The model under review builds one solid part; all positions refer to its coordinate system, in mm. A direction names the side the tool comes from. Round coordinates to 2 decimals unless told otherwise and drop trailing zeros. Loops run counter-clockwise (first coordinate to the right, second up) from the corner with the lowest first, then second, coordinate; pieces in that order, holes last. Notation, with made-up numbers: (51.5, -16) -> (55.5, -16) arc R24 ccw to (55.5, 23) -> close; hole circle Ø6 at (57, -12). An arc over 180 degrees is marked (long way). Use a Markdown table: item, result. Add a question column.
1) Mouldability with a two-part tool opening along Z and no side actions: class faces 5 (the cylindrical face through (8.728, 9.028, -60.264)), 6 (the cylindrical face through (5, 2, 0)), 7 (the cylindrical face through (19.014, 16.377, -42.653)) as released by +Z, released by -Z, zero draft, split by the parting line, or undercut.
2) Consider section B-B on x = 12.7. Give the boundary of the cut face in (y, z) (3 decimals), plus the area to 3 significant figures.
3) Consider section A-A on z = 8.75. Give the boundary of the cut face in (x, y).
4) Wall thickness on probe 1 along X at (y, z) = (10.5, -55); probe 2 along X at (y, z) = (12.25, -1.5); probe 3 along Y at (x, z) = (-12.7, -55.5) (3 decimals): over which ranges is each line inside the solid? List them lowest first.
5) Consider section C-C on z = -32.5. Give the boundary of the cut face in (x, y), plus the area to 3 significant figures.
6) Consider section D-D on x = 5. State how many separate pieces and enclosed holes the cut face has, plus the area to 3 significant figures.
7) Insertion check: pin 1 (1 mm diameter, centred on x = -15.5, z = -24, fed in from +Y); pin 2 (2 mm diameter, centred on x = 14, y = 17.5, fed in from +Z); pin 3 (4.5 mm diameter, centred on x = -2.5, y = 2, fed in from -Z); pin 4 (8 mm diameter, centred on x = -4.5, z = -44, fed in from +Y). Each pin has a flat end and moves straight along its axis. Give the tip position at first contact, or say it passes through.
8) For faces 1 (the flat face through (19, 15, 13)), 2 (the flat face through (0, 14.175, -56)), 3 (the cylindrical face through (-15.27, 2.46, -22.47)), 4 (the flat face through (13, 5, 10)), list the 3-axis set-ups (+Z, -Z, +X, -X, +Y, -Y) from which the entire face can be reached by the end or side of a thin tool; tool diameter is ignored.
from build123d import *

# Parameters (mm, degrees)
MAIN_DEPTH                      = 61.25
FRONT_CONGE_R                   = 3
ESQUISSE11_W                    = 2
ESQUISSE11_H                    = 15
DSUB_EXTRUSION_ATTACHMENT_DEPTH = 15
ESQUISSE12_W                    = 40
ESQUISSE12_H                    = 15
ESQUISSE12_R                    = 1.35
ESQUISSE12_W_2                  = 16
ESQUISSE12_H_2                  = 7
DSUB_EXTRUSION_DEPTH            = 15
DSUB_FRONT_HOLE_DEPTH           = 5.5
ESQUISSE14_R                    = 4.3
BOTTOM_HOLE_DEPTH               = 2
SKETCH7_W                       = 36
SKETCH7_H                       = 10
DSUBBOTTOMHOLE_DEPTH            = 1
CONG_4_R                        = 10
BOTTOMSTOP_REACH                = 77.839
SKETCH4_W                       = 6.5
SKETCH4_H                       = 7
FILLET1_R                       = 1
SKETCH5_W                       = 16
SKETCH5_H                       = 12
CUT_EXTRUDE1_DEPTH              = 14.175
SKETCH6_R                       = 1.25
FIXHOLE_DEPTH                   = 68.465268843
LPATTERN1_COUNT                 = 8
LPATTERN1_PITCH                 = 10
LPATTERN1_COUNT_DIR2            = 4
LPATTERN1_PITCH_DIR2            = 10


with BuildPart() as part:
    # Esquisse1 → Main (new, symmetric)
    with BuildSketch(Plane.XY):
        Polygon((18, 15), (20, 15), (20, 0), (-20, 0), (-20, 15), (-18, 15), (-18, 5), (-8, 5), (-8, 4), (8, 4), (8, 5), (18, 5), align=None)
    extrude(amount=MAIN_DEPTH, both=True)

    # Front Conge
    # the kernel refuses this fillet: 3 mm, written as the material it takes off along each edge
    with BuildSketch(Plane(origin=(18, 5, 61.25), x_dir=(1, 0, 0), z_dir=(0, 1, 0)), Plane(origin=(-18, 22.071067812, 61.25), x_dir=(-1, 0, 0), z_dir=(0, -1, 0))) as front_conge_piece_1:
        with BuildLine():
            CenterArc((3, 2.828427125), FRONT_CONGE_R, 180, 70.528779366)
            Line((0, 2.828427125), (-0.06, 2.828427125))
            Line((-0.06, 2.828427125), (-0.06, 0))
            Line((-0.06, 0), (0, -0.06))
            ThreePointArc((0, -0.06), (1, -0.06), (1.98, -0.056568542))
            Line((1.98, -0.056568542), (2, 0))
        make_face()
    extrude(amount=17.071067812, mode=Mode.SUBTRACT)

    # Esquisse11 → DSub-Extrusion Attachment (add)
    with BuildSketch(Plane(origin=(0, 0, -46.25), x_dir=(-1, 0, 0), z_dir=(0, 0, -1))):
        with Locations((-19, 12.5)):
            Rectangle(ESQUISSE11_W, ESQUISSE11_H)
        with Locations((19, 12.5)):
            Rectangle(ESQUISSE11_W, ESQUISSE11_H)
    extrude(amount=DSUB_EXTRUSION_ATTACHMENT_DEPTH)

    # Esquisse12 → DSub-Extrusion (add)
    with BuildSketch(Plane(origin=(0, 0, -46.25), x_dir=(-1, 0, 0), z_dir=(0, 0, -1))):
        with Locations((0, 12.5)):
            Rectangle(ESQUISSE12_W, ESQUISSE12_H)
        with Locations((-12.7, 10.675)):
            Circle(ESQUISSE12_R, mode=Mode.SUBTRACT)
        with Locations((12.7, 10.675)):
            Circle(ESQUISSE12_R, mode=Mode.SUBTRACT)
        with Locations((0, 10.675)):
            Rectangle(ESQUISSE12_W_2, ESQUISSE12_H_2, mode=Mode.SUBTRACT)
    extrude(amount=DSUB_EXTRUSION_DEPTH)

    # Esquisse13 → DSub-Front Hole (cut)
    with BuildSketch(Plane.XY.offset(-46.25)):
        Polygon((-10, 17), (10, 17), (8.5, 5), (-8.5, 5), align=None)
    extrude(amount=-DSUB_FRONT_HOLE_DEPTH, mode=Mode.SUBTRACT)

    # Esquisse14 → Bottom Hole (cut)
    with BuildSketch(Plane(origin=(0, 0, -61.25), x_dir=(-1, 0, 0), z_dir=(0, 0, -1))):
        with Locations((-12.7, 10.675)):
            Circle(ESQUISSE14_R)
        with Locations((12.7, 10.675)):
            Circle(ESQUISSE14_R)
    extrude(amount=-BOTTOM_HOLE_DEPTH, mode=Mode.SUBTRACT)

    # Sketch7 → DSubBottomHole (cut)
    with BuildSketch(Plane(origin=(0, 5, 0), x_dir=(1, 0, 0), z_dir=(0, 1, 0))):
        with Locations((0, 41.25)):
            Rectangle(SKETCH7_W, SKETCH7_H)
    extrude(amount=-DSUBBOTTOMHOLE_DEPTH, mode=Mode.SUBTRACT)

    # Congé4
    # the kernel refuses this fillet: 10 mm, written as the material it adds along each edge
    with BuildSketch(Plane(origin=(-18, 15, -46.25), x_dir=(0, 1, 0), z_dir=(-1, 0, 0)), Plane(origin=(20, 15, -46.25), x_dir=(0, 1, 0), z_dir=(-1, 0, 0))) as cong_4_piece_1:
        with BuildLine():
            CenterArc((10, -8.660254038), CONG_4_R, 120, 60)
            Line((0, -8.660254038), (0, 0))
            Line((0, 0), (5, 0))
        make_face()
    extrude(amount=2)

    # BottomStop: up to this face of the body (flat: up to its plane)
    bottomstop_end = Plane(part.part.faces().sort_by_distance((20, 7.947826544, -2.383218252))[0])
    # Sketch4 → BottomStop (add, up to the picked face)
    with BuildSketch(Plane.ZY.offset(20), mode=Mode.PRIVATE) as bottomstop_sk1:
        with Locations((58, 3.5)):
            Rectangle(SKETCH4_W, SKETCH4_H)
    bottomstop_tool1 = split(extrude(bottomstop_sk1.sketch, amount=-BOTTOMSTOP_REACH, mode=Mode.PRIVATE), bisect_by=bottomstop_end, keep=Keep.BOTH, mode=Mode.PRIVATE)
    add(bottomstop_tool1.solids().sort_by(Axis((-20, 3.5, 58), (1, 0, 0)))[0])

    # Fillet1
    fillet1_edges = [part.edges().sort_by_distance(p)[0] for p in [
        (0, 4, 54.75),
        (0, 7, 54.75),
    ]]
    fillet(fillet1_edges, radius=FILLET1_R)

    # Sketch5 → Cut-Extrude1 (cut)
    with BuildSketch(Plane(origin=(0, 0, 0), x_dir=(-1, 0, 0), z_dir=(0, -1, 0))):
        with Locations((0, 55.25)):
            Rectangle(SKETCH5_W, SKETCH5_H)
    extrude(amount=-CUT_EXTRUDE1_DEPTH, mode=Mode.SUBTRACT)

    # Sketch6 → FixHole (cut, through all)
    with BuildSketch(Plane(origin=(0, 0, 0), x_dir=(-1, 0, 0), z_dir=(0, -1, 0))):
        with Locations(Location((15, -48.75, 0), (0, 0, 180))):
            Circle(SKETCH6_R)
    fixhole = extrude(amount=-FIXHOLE_DEPTH, mode=Mode.SUBTRACT)

    # LPattern1: FixHole 8 × 4
    with Locations(*[(j * LPATTERN1_PITCH_DIR2, 0, -i * LPATTERN1_PITCH) for i in range(LPATTERN1_COUNT) for j in range(LPATTERN1_COUNT_DIR2) if (i, j) != (0, 0)]):
        add(fixhole, mode=Mode.SUBTRACT)


solid = part.part
Result set:
| question | item | result |
|---|---|---|
| 1 | face 5 | zero draft |
| 1 | face 6 | undercut |
| 1 | face 7 | released by +Z |
| 2 | outline | (0, -61.25) -> (6.375, -61.25) -> (6.375, -59.25) -> (9.325, -59.25) -> (9.325, -46.25) -> (4, -46.25) -> (4, -36.25) -> (5, -36.25) -> (5, 54.75) -> (6, 54.75) arc R1 ccw to (7, 55.75) -> (7, 61.25) -> (0, 61.25) -> close; (12.025, -59.25) -> (14.975, -59.25) -> (14.975, -61.25) -> (20, -61.25) -> (20, -46.25) -> (12.025, -46.25) -> close |
| 2 | area | 788 mm2 |
| 3 | outline | (-20, 0) -> (-16.25, 0) -> (-16.25, 5) -> (-18, 5) -> (-18, 15) -> (-20, 15) -> close; (-13.75, 0) -> (-6.25, 0) -> (-6.25, 4) -> (-8, 4) -> (-8, 5) -> (-13.75, 5) -> close; (-3.75, 0) -> (3.75, 0) -> (3.75, 4) -> (-3.75, 4) -> close; (6.25, 0) -> (13.75, 0) -> (13.75, 5) -> (8, 5) -> (8, 4) -> (6.25, 4) -> close; (16.25, 0) -> (20, 0) -> (20, 15) -> (18, 15) -> (18, 5) -> (16.25, 5) -> close |
| 4 | probe 1 | -20 to -14.04, -11.36 to -8, 8 to 11.36, 14.04 to 20 |
| 4 | probe 2 | -20 to -18, 18 to 20 |
| 4 | probe 3 | 0 to 9.325, 12.025 to 20 |
| 5 | outline | (-20, 0) -> (20, 0) -> (20, 15) -> (18, 15) -> (18, 5) -> (8, 5) -> (8, 4) -> (-8, 4) -> (-8, 5) -> (-18, 5) -> (-18, 15) -> (-20, 15) -> close |
| 5 | area | 224 mm2 |
| 6 | separate pieces | 10 |
| 6 | enclosed holes | 0 |
| 6 | area | 453 mm2 |
| 7 | pin 1 | y = 5 |
| 7 | pin 2 | z = -46.25 |
| 7 | pin 3 | z = -49.25 |
| 7 | pin 4 | y = 20 |
| 8 | face 1 | +Z, +X, -X, +Y |
| 8 | face 2 | +Z, -Z, -Y |
| 8 | face 3 | +Y, -Y |
| 8 | face 4 | +Y |
